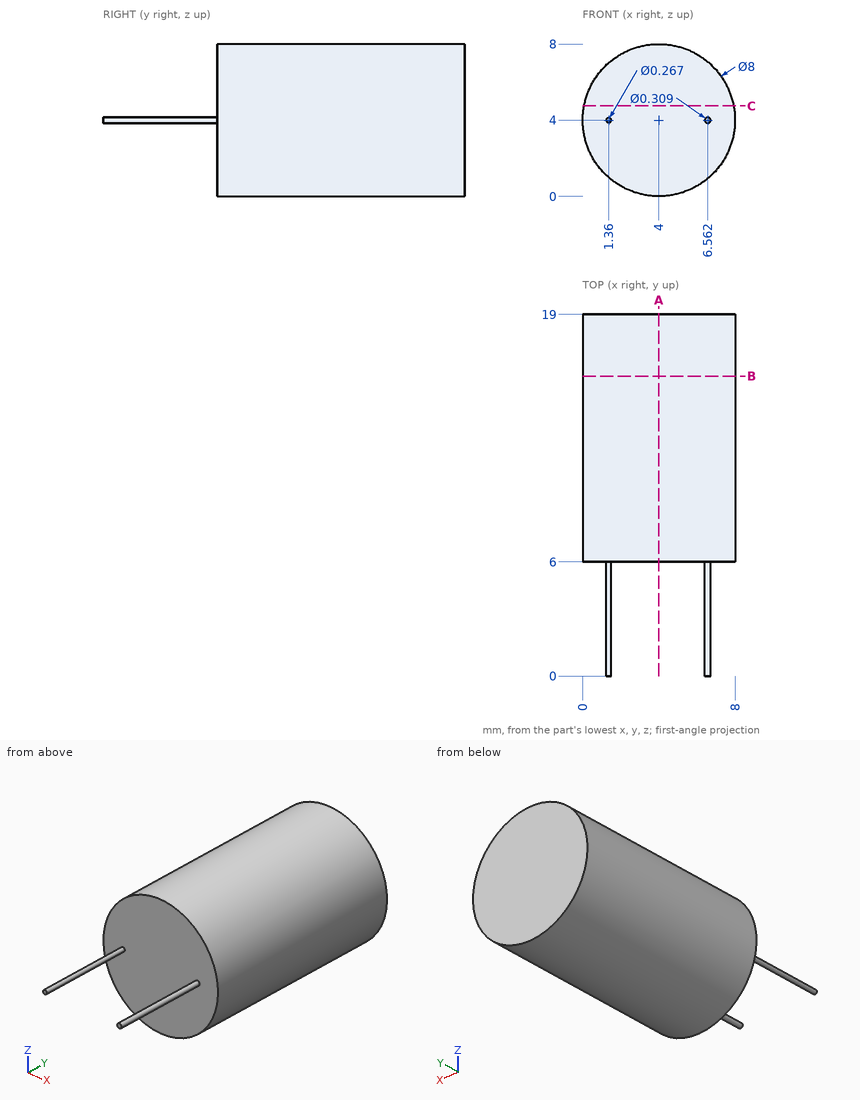
Study the drawing (mm; zero at the part's minimum x, y, z) and answer. Round coordinates to 2 decimals unless told otherwise and drop trailing zeros. Write each loop counter-clockwise with the first axis right and the second up, starting at its lowest first coordinate (ties: lowest second). Pieces come first, ordered by that corner, then holes. Notation, with made-up numbers: (73.5, 24.25) - (82.5, 24.25) arc R29 ccw to (82.5, 47.25) - close; hole circle Ø5 at (0.25, -23). An arc over 180 degrees is marked (long way). Return JSON: item names as keys, results as strings. Group by question number.
Q1. Find the intervals of material crossed by L1, parallel to Y at x = 4.25, z = 3; L2, parallel to Z at x = 1.25, y = 13 (1 decimal); L3, parallel to X at y = 16, z = 5.5, in increasing order.
Q2. The part is cut by section C-C on z = 4.75. Write down the section's boundary in (x, y).
Q3. This flat-tipped pin is pushed along its axis until it touches: pin 1 Ø4 at (x, z) = (4.5, 2.5) entering from -Y. Where does it stop, or does it pass through?
Q4. The part is cut by section B-B on y = 15.75. Write down the section's boundary in (x, z).
Q5. The part is cut by section A-A on x = 4. Write down the section's boundary in (y, z), then the cut area to 3 significant figures.
Solved:
{
 "1": {"L1": "6 to 19", "L2": "1.1 to 6.9", "L3": "0.29 to 7.71"},
 "2": {"outline": "(0.07, 6) - (7.93, 6) - (7.93, 19) - (0.07, 19) - close"},
 "3": {"pin 1": "y = 6"},
 "4": {"outline": "circle Ø8 at (4, 4)"},
 "5": {"outline": "(6, 0) - (19, 0) - (19, 8) - (6, 8) - close", "area": "104 mm²"}
}
